Design review of the part built by this model. Coordinates are the model's own, in mm. Face numbers are marked on the shaded views. A direction names the side the tool comes from. Coordinates: 2 decimals unless noted, no trailing zeros. Write each loop counter-clockwise with the first axis right and the second up, starting at its lowest first coordinate (ties: lowest second). Pieces come first, ordered by that corner, then holes. Notation, with made-up numbers: (-25.75, -34.75) - (-12.75, -34.75) arc R16 ccw to (-12.75, -19.75) - close; hole circle Ø2 at (57.25, -10). An arc over 180 degrees is marked (long way). Answer as CSV lines item,"result". Start each with the question number.
Q1. We need section B-B (y = 120). Write out the cut boundary in (x, z).
Q2. We need section A-A (z = -47). Write out the cut boundary in (x, y), plus the area to 3 significant figures.
Q3. For line 1 along Z through (x, y) = (-46, 354); line 2 along X through (y, z) = (268, 12.5); line 3 along Y through (x, z) = (-194.5, 157.5), list the stretches that pass through material, from the lowest coordinate up. Write a range as [from, to].
Q4. Machinability: for the marked faces 4 and 5, which of the approach directions +Z, -Z, +X, -X, +Y, -Y give a long, thin tool a straight path to every point of the face, cutting with its end or side? Answer none if there is none.
Q5. Clearance check with a flat-ended pin moving along its axis: pin 1 (3 mm diameter, centred on x = -318, z = -11, fed in from +Y). State where the tip first meets the part, or that it passes through.
Q6. Mouldability with a two-part tool opening along Z and no side actions: class the marked faces 1, 2 and 3 as pulls with the +Z half, pulls with the -Z half, needs draft (parallel to the pull), parting line crosses it, or undercut.
Q7. We need section C-C (x = 90.5). Write out the cut boundary in (y, z), plus the area to 3 significant figures.
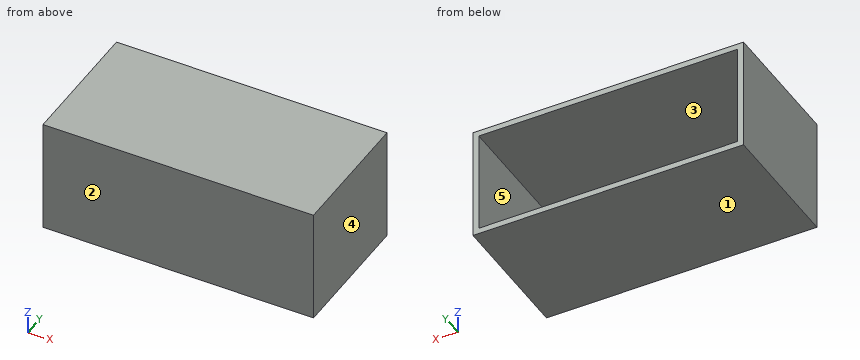
from build123d import *

# Parameters (mm, degrees)
SKETCH1_W          = 929
SKETCH1_H          = 392
BOTTOM_PLATE_DEPTH = 20
SKETCH2_W          = 929
SKETCH2_H          = 20
LEFT_WALL_DEPTH    = 462
SKETCH3_W          = 929
SKETCH3_H          = 20
RIGHT_WALL_DEPTH   = 462
SKETCH4_W          = 20
SKETCH4_H          = 352
BACK_WALL_DEPTH    = 462
SKETCH5_W          = 20
SKETCH5_H          = 352
FRONT_WALL_DEPTH   = 462


with BuildPart() as part:
    # Sketch1 → Bottom Plate (new body)
    with BuildSketch(Plane(origin=(0, 0, 0), x_dir=(1, 0, 0), z_dir=(0, 1, 0))):
        Rectangle(SKETCH1_W, SKETCH1_H)
    extrude(amount=BOTTOM_PLATE_DEPTH)

    # Sketch2 → Left Wall (add)
    with BuildSketch(Plane(origin=(0, 0, 0), x_dir=(1, 0, 0), z_dir=(0, 1, 0))):
        with Locations((0, 186)):
            Rectangle(SKETCH2_W, SKETCH2_H)
    extrude(amount=LEFT_WALL_DEPTH)

    # Sketch3 → Right Wall (add)
    with BuildSketch(Plane(origin=(0, 0, 0), x_dir=(1, 0, 0), z_dir=(0, 1, 0))):
        with Locations((0, -186)):
            Rectangle(SKETCH3_W, SKETCH3_H)
    extrude(amount=RIGHT_WALL_DEPTH)

    # Sketch4 → Back Wall (add)
    with BuildSketch(Plane(origin=(0, 0, 0), x_dir=(1, 0, 0), z_dir=(0, 1, 0))):
        with Locations((454.5, 0)):
            Rectangle(SKETCH4_W, SKETCH4_H)
    extrude(amount=BACK_WALL_DEPTH)

    # Sketch5 → Front Wall (add)
    with BuildSketch(Plane(origin=(0, 0, 0), x_dir=(1, 0, 0), z_dir=(0, 1, 0))):
        with Locations((-454.5, 0)):
            Rectangle(SKETCH5_W, SKETCH5_H)
    extrude(amount=FRONT_WALL_DEPTH)


solid = part.part
Results list:
1,outline,"(-464.5, -196) - (464.5, -196) - (464.5, 196) - (-464.5, 196) - close; hole (-444.5, -176) - (444.5, -176) - (444.5, 176) - (-444.5, 176) - close"
2,outline,"(-464.5, 0) - (464.5, 0) - (464.5, 462) - (444.5, 462) - (444.5, 20) - (-444.5, 20) - (-444.5, 462) - (-464.5, 462) - close"
2,area,"36,300 mm2"
3,line 1,"z = [-196, -176], [176, 196]"
3,line 2,"x = [-464.5, -444.5], [444.5, 464.5]"
3,line 3,"y = [0, 20]"
4,face 4,"+Z, -Z, +X, +Y, -Y"
4,face 5,"+Y"
5,pin 1,"stops at y = 20"
6,face 1,"pulls with the -Z half"
6,face 2,"needs draft"
6,face 3,"undercut"
7,outline,"(0, -196) - (462, -196) - (462, -176) - (20, -176) - (20, 176) - (462, 176) - (462, 196) - (0, 196) - close"
7,area,"25,500 mm2"
